Input: part model. Units: mm. Frame: model coordinates. A direction names the side the tool comes from. Coordinates: 2 decimals unless noted, no trailing zeros. Order: outer loops, then holes, each group sorted by start corner. A loop starts at its lowest first (then second) coordinate and runs counter-clockwise, first axis right, second up. Notation, with made-up numbers: (45, -38) - (56, -38) arc R24 cw to (56, -10) - close; hole circle Ø4 at (69.5, 1.5). An arc over 180 degrees is marked (long way). Use a Markdown table: item, result. Add a question column.
Autodesk Inventor part; units mm, degrees
ref_plane "YZ Plane" through (0, 0, 0) normal (1, 0, 0) x (0, 1, 0)
ref_plane "XZ Plane" through (0, 0, 0) normal (0, 1, 0) x (-1, 0, 0)
ref_plane "XY Plane" through (0, 0, 0) normal (0, 0, 1) x (1, 0, 0)
sketch "Sketch1" plane through (0, 0, 0) normal (0, 1, 0) x (-1, 0, 0)
  line L0 (-90.5, 80) -> (90.5, 80) construction
  line L1 (90.5, 80) -> (90.5, -80) construction
  line L2 (90.5, -80) -> (-90.5, -80) construction
  line L3 (-90.5, -80) -> (-90.5, 80) construction
  line L4 (-90.5, 80) -> (90.5, -80) construction
  line L5 (90.5, 80) -> (-90.5, -80) construction
  circle A0 centre (90.5, 80) radius 1.65
  circle A1 centre (90.5, -80) radius 1.65
  circle A2 centre (-90.5, -80) radius 1.65
  circle A3 centre (-90.5, 80) radius 1.65
  line L6 (97.5, 120) -> (-97.5, 120)
  line L7 (-97.5, 120) -> (-97.5, -170)
  line L8 (-97.5, -170) -> (97.5, -170)
  line L9 (97.5, -170) -> (97.5, 120)
  line L10 (80, 120) -> (80, -170)
  line L11 (0, 0) -> (0, -42.6616)
  line L12 (-80, 120) -> (-80, -170)
  line L13 (-97.5, -93) -> (97.5, -93)
  point P0 (0, -170)
  point P1 (-80, -93)
  point P2 (80, -93)
  dimension "d0" = 181
  dimension "d1" = 160
  dimension "d2" = 3.3
  dimension "d3" = 40
  dimension "d4" = 290
  dimension "d5" = 7
  dimension "d7" = 10.5
  dimension "d8" = 13
extrude "Extrusion1" add sketch "Sketch1" along normal blind 7.5 contours L9 L13 L10 L6 | L12 L13 L7 L6
extrude "Extrusion2" add sketch "Sketch1" against normal blind 1 contours L9 L13 L10 L6 | L9 L8 L10 L13 | L12 L13 L7 L6 | L12 L8 L7 L13
sketch "Sketch2" plane through (0, -1, 0) normal (0, -1, 0) x (1, 0, 0)
  line L0 (97.5, 120) -> (80, 120)
  line L1 (80, 120) -> (80, -170)
  line L2 (80, -170) -> (97.5, -170)
  line L3 (97.5, -170) -> (97.5, 120)
  circle A0 centre (90.5, 80) radius 1.65
  circle A1 centre (90.5, -80) radius 1.65
  line L4 (-97.5, -170) -> (-80, -170)
  line L5 (-80, -170) -> (-80, 120)
  line L6 (-80, 120) -> (-97.5, 120)
  line L7 (-97.5, 120) -> (-97.5, -170)
  circle A2 centre (-90.5, -80) radius 1.65
  circle A3 centre (-90.5, 80) radius 1.65
  line L8 (-80, -170) -> (80, -170)
  line L9 (80, -170) -> (80, 120)
  line L10 (80, 120) -> (-80, 120)
  line L11 (-80, 120) -> (-80, -170)
  line L12 (-80, -170) -> (-85, -170)
  line L13 (-85, -170) -> (-85, 120)
  line L14 (-85, 120) -> (-80, 120)
  line L15 (-80, 120) -> (-80, -170)
  line L16 (-70, -170) -> (70, -170)
  line L17 (70, -170) -> (70, 120)
  line L18 (70, 120) -> (-70, 120)
  line L19 (-70, 120) -> (-70, -170)
  line L20 (0, 0) -> (0, 25.7768)
  line L21 (85, -170) -> (85, 120)
  point P0 (0, 120)
  point P1 (85, 120)
  dimension "d13" = 5
  dimension "d14" = 140
extrude "Extrusion3" add sketch "Sketch2" along normal blind 5 contours L21 L2 L1 L0 | L1 L8 L17 L10 | L19 L8 L5 L10 | L5 L4 L13 L6
sketch "Sketch3" plane through (0, -6, 0) normal (0, -1, 0) x (1, 0, 0)
  line L0 (-85, -170) -> (-70, -170)
  line L1 (-70, -170) -> (-70, 120)
  line L2 (-70, 120) -> (-85, 120)
  line L3 (-85, 120) -> (-85, -170)
  line L4 (85, 120) -> (70, 120)
  line L5 (70, 120) -> (70, -170)
  line L6 (70, -170) -> (85, -170)
  line L7 (85, -170) -> (85, 120)
  line L8 (-70, -170) -> (70, -170)
  line L9 (70, -170) -> (70, 120)
  line L10 (70, 120) -> (-70, 120)
  line L11 (-70, 120) -> (-70, -170)
  line L12 (65, -165) -> (-65, -165)
  line L13 (-65, -165) -> (-65, 115)
  line L14 (-65, 115) -> (65, 115)
  line L15 (65, 115) -> (65, -165)
  point P0 (0, 0)
  dimension "d19" = 140
  dimension "d20" = 290
  dimension "d21" = 5
extrude "Extrusion4" add sketch "Sketch3" along normal blind 100 and the other way blind 5 contours L1 L10 L5 L8
fillet "Fillet1" radius 6 2 edges at (80, 7.5, 13.5) (-80, 7.5, 13.5)
chamfer "Chamfer1" distance 10 angle 45 2 edges at (70, -6, -25) (-70, -6, -25)
chamfer "Chamfer2" distance 5 angle 45 2 edges at (-65, -1, -25) (65, -1, -25)
chamfer "Chamfer3" distance 2.5 angle 45 2 edges at (-85, -1, -25) (-85, -6, -25)
sketch "Sketch4" plane through (97.5, -1, 120) normal (0, 0, 1) x (1, 0, 0)
  line L0 (-180, -5) -> (-185, 0)
  line L1 (-177.5, -5) -> (-180, -5)
  line L2 (-167.5, -15) -> (-177.5, -5)
  line L3 (-167.5, -105) -> (-167.5, -15)
  line L4 (-27.5, -105) -> (-167.5, -105)
  line L5 (-27.5, -15) -> (-27.5, -105)
  line L6 (-17.5, -5) -> (-27.5, -15)
  line L7 (-12.5, -5) -> (-17.5, -5)
  line L8 (-12.5, 0) -> (-12.5, -5)
  line L9 (0, 0) -> (-12.5, 0)
  line L10 (0, 0) -> (0, 8.5)
  line L11 (-11.5, 8.5) -> (0, 8.5)
  arc A0 (-11.5, 8.5) -> (-17.5, 2.5) centre (-11.5, 2.5) ccw
  line L12 (-17.5, 0) -> (-17.5, 2.5)
  line L13 (-17.5, 0) -> (-177.5, 0)
  line L14 (-177.5, 0) -> (-177.5, 2.5)
  arc A1 (-177.5, 2.5) -> (-183.5, 8.5) centre (-183.5, 2.5) ccw
  line L15 (-195, 8.5) -> (-183.5, 8.5)
  line L16 (-195, 0) -> (-195, 8.5)
  line L17 (-185, 0) -> (-195, 0)
  circle A2 centre (-97.5, -105) radius 81
  line L18 (-107.5, 0) -> (-87.5, 0)
  line L19 (-87.5, 0) -> (-87.5, -15)
  line L20 (-87.5, -15) -> (-107.5, -15)
  line L21 (-107.5, -15) -> (-107.5, 0)
  point P0 (-97.5, 1)
  point P1 (-97.5, 0)
  point P2 (-97.5, -15)
  point P3 (-97.5, 0)
  point P4 (-27.5, -64.2446)
  point P5 (-167.5, -64.2446)
  dimension "d36" = 15
  dimension "d37" = 20
  dimension "d40" = 162
extrude "Extrusion5" cut sketch "Sketch4" against normal through all contours A2 L5 L4 L3 | L13 L19 L20 L21 picked at (-97.5, -78)
properties part number "PUERTA_ACOPLE_ENTRADA" material "Steel, Mild, Welded"
1) Cut plane C-C (y = -46). Return the cut outline in (x, z), and give its area (3 significant figures).
2) Cut plane A-A (y = -11). Return the cut outline in (x, z).
3) Contact query for flat-ended pins moving along their axis: P1, Ø4, axis at y = -46.5, z = -128, coming from the -X side; P2, Ø2.5, axis at y = -11, z = 118.5, coming from the -X side; P3, Ø2, axis at x = 90.5, z = 80, coming from the +Y side; P4, Ø12, axis at y = -18.5, z = 51.5, coming from the +X side. Output: stop coordinate, or through.
4) Material intervals for L1, parallel to Z at x = -90.5, y = 5.25; L2, parallel to X at y = 0.75, z = 80; L3, parallel to Z at x = -43.5, y = -31, sorted ascending.
5) Reachability of faces 1 (the flat face through (91, -1, -23)), 2 (the flat face through (-71, -1, -3)), 3 (the flat face through (-65, -31, -27)), 4 (the flat face through (-70, -40, -27)) from +Z, -Z, +X, -X, +Y, -Y: full face, straight path, thin tool, end or side. Return the list, or none.
6) Pull-direction query (Z, two-part tool) for faces 5 (the flat face through (-97.5, 3, 5)), 6 (the flat face through (65, -31, -23)), 7 (the flat face through (1, -18, -170)); classes: pulls with the +Z half, pulls with the -Z half, needs draft (parallel to the pull), parting line crosses it, or undercut.
Computed:
| question | item | result |
|---|---|---|
| 1 | outline | (-70, -170) - (-54.42, -170) - (-54.42, -165) - (-65, -165) - (-65, 115) - (-54.42, 115) - (-54.42, 120) - (-70, 120) - close; (54.42, -170) - (70, -170) - (70, 120) - (54.42, 120) - (54.42, 115) - (65, 115) - (65, -165) - (54.42, -165) - close |
| 1 | area | 3,110 mm2 |
| 2 | outline | (-75, -170) - (-10, -170) - (-10, -165) - (-65, -165) - (-65, 115) - (-10, 115) - (-10, 120) - (-75, 120) - close; (10, -170) - (75, -170) - (75, 120) - (10, 120) - (10, 115) - (65, 115) - (65, -165) - (10, -165) - close |
| 3 | P1 | stops at x = -70 |
| 3 | P2 | stops at x = -76.25 |
| 3 | P3 | passes through |
| 3 | P4 | stops at x = 73.5 |
| 4 | L1 | z = -93 to -81.65, -78.35 to 78.35, 81.65 to 120 |
| 4 | L2 | x = -97.5 to -92.15, -88.85 to -80, 80 to 88.85, 92.15 to 97.5 |
| 4 | L3 | z = -170 to -165, 115 to 120 |
| 5 | face 1 | +Z, -Z, +X, -Y |
| 5 | face 2 | +Z, -Z, +Y |
| 5 | face 3 | +Y, -Y |
| 5 | face 4 | +Z, -Z, -X, -Y |
| 6 | face 5 | needs draft |
| 6 | face 6 | undercut |
| 6 | face 7 | pulls with the -Z half |
